Input: part model. Units: mm. Frame: model coordinates. Face numbers are marked on the shaded views. A direction names the side the tool comes from. Round coordinates to 2 decimals unless told otherwise and drop trailing zeros. Order: outer loops, then holes, each group sorted by start corner. A loop starts at its lowest first (then second) coordinate and runs counter-clockwise, first axis right, second up. Notation, with made-up numbers: M -6.5,-31.5 L 50.5,-31.5 A30 ccw 50.5,7.5 Z; hole C 46,17.25 d2. An arc over 180 degrees is marked long. One line per question, with ' | ' between items.
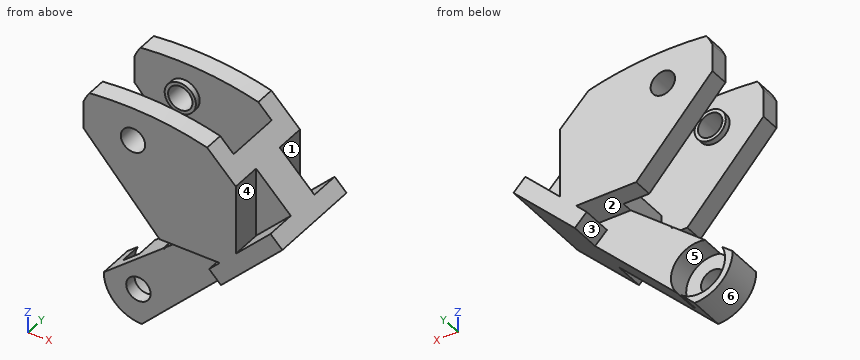
```python
from build123d import *

# Parameters (mm, degrees)
SKETCH_1_R           = 1.6
EXTRUDE_1_DEPTH      = 4.65
SKETCH_7_W           = 9
SKETCH_7_H           = 19
EXTRUDE_4_DEPTH      = 4
SKETCH_8_W           = 9
SKETCH_8_H           = 19
EXTRUDE_5_DEPTH      = 4
SKETCH_9_W           = 16
SKETCH_9_H           = 7.5
CUT_EXTRUDE_3_DEPTH  = 9
SKETCH_11_R          = 1.6
CUT_EXTRUDE_5_DEPTH  = 26.4
EXTRUDE_6_DEPTH      = 9
SKETCH_13_W          = 19
SKETCH_13_H          = 12.65
EXTRUDE_7_DEPTH      = 2
SKETCH_15_W          = 7.596607022
SKETCH_15_H          = 7.5
CUT_EXTRUDE_6_DEPTH  = 8
CUT_EXTRUDE_7_DEPTH  = 8
EXTRUDE_8_DEPTH      = 4.65
CUT_EXTRUDE_9_DEPTH  = 4.65
SKETCH_20_W          = 5.380169682
SKETCH_20_H          = 3
CUT_EXTRUDE_10_DEPTH = 7.5
CUT_EXTRUDE_11_DEPTH = 4.65
CUT_EXTRUDE_13_DEPTH = 13
CUT_EXTRUDE_15_DEPTH = 13
SKETCH_26_W          = 18.396488504
SKETCH_26_H          = 12.65
EXTRUDE_9_DEPTH      = 2.2
SKETCH_28_W          = 2.5
SKETCH_28_H          = 12.65
CUT_EXTRUDE_17_DEPTH = 18
CUT_EXTRUDE_18_DEPTH = 14
SKETCH_31_W          = 5
SKETCH_31_H          = 12.65
CUT_EXTRUDE_19_DEPTH = 20
SKETCH_32_R          = 3.55
CUT_EXTRUDE_20_DEPTH = 3
EXTRUDE_START        = 0.75
SKETCH_33_R          = 2.05
SKETCH_33_R_2        = 1.6
EXTRUDE_10_DEPTH     = 0.75
SKETCH_34_R          = 2.05
SKETCH_34_R_2        = 1.6
EXTRUDE_11_DEPTH     = 0.75


with BuildPart() as part:
    # 草图1 → 凸台-拉伸1 (new body)
    with BuildSketch(Plane(origin=(0, 0, 0), x_dir=(1, 0, 0), z_dir=(0, 1, 0))):
        with BuildLine():
            Line((5, 0), (20, 0))
            Line((20, 0), (20, -16))
            Line((20, -16), (9, -16))
            Line((9, -16), (9, -35))
            Line((9, -35), (0, -35))
            Line((0, -35), (0, -27))
            Line((0, -27), (0, -5))
            ThreePointArc((0, -5), (1.464466094, -1.464466094), (5, 0))
        make_face()
        with Locations(Location((4.55, -4.55, 0), (0, 0, 270))):
            Circle(SKETCH_1_R, mode=Mode.SUBTRACT)
    extrude(amount=EXTRUDE_1_DEPTH)

    # 草图7 → 凸台-拉伸4 (add)
    with BuildSketch(Plane(origin=(0, 4.65, 0), x_dir=(1, 0, 0), z_dir=(0, 1, 0))):
        with Locations((4.5, -25.5)):
            Rectangle(SKETCH_7_W, SKETCH_7_H)
    extrude(amount=EXTRUDE_4_DEPTH)

    # 草图8 → 凸台-拉伸5 (add)
    with BuildSketch(Plane.XZ):
        with Locations((4.5, 25.5)):
            Rectangle(SKETCH_8_W, SKETCH_8_H)
    extrude(amount=EXTRUDE_5_DEPTH)

    # 草图9 → 切除-拉伸3 (cut)
    with BuildSketch(Plane.ZY):
        with Locations((27, 2.325)):
            Rectangle(SKETCH_9_W, SKETCH_9_H)
    extrude(amount=-CUT_EXTRUDE_3_DEPTH, mode=Mode.SUBTRACT)

    # 草图11 → 切除-拉伸5 (cut)
    with BuildSketch(Plane(origin=(0, 8.65, 0), x_dir=(1, 0, 0), z_dir=(0, 1, 0))):
        with Locations(Location((6.5, -28, 0), (0, 0, 270))):
            Circle(SKETCH_11_R)
    extrude(amount=-CUT_EXTRUDE_5_DEPTH, mode=Mode.SUBTRACT)

    # 草图12 → 凸台-拉伸6 (add)
    with BuildSketch(Plane(origin=(9, 0, 0), x_dir=(0, 0, -1), z_dir=(1, 0, 0))):
        Polygon((-35, 8.65), (-35, 6.075), (-19, 6.075), (-19, -1.425), (-35, -1.425), (-35, -4), (-16, -4), (-16, 8.65), align=None)
    extrude(amount=EXTRUDE_6_DEPTH)

    # 草图13 → 凸台-拉伸7 (add)
    with BuildSketch(Plane(origin=(18, 0, 0), x_dir=(0, 0, -1), z_dir=(1, 0, 0))):
        with Locations((-25.5, 2.325)):
            Rectangle(SKETCH_13_W, SKETCH_13_H)
    extrude(amount=EXTRUDE_7_DEPTH)

    # 草图15 → 切除-拉伸6 (cut)
    with BuildSketch(Plane.ZY):
        with Locations((15.201696489, 2.325)):
            Rectangle(SKETCH_15_W, SKETCH_15_H)
    extrude(amount=-CUT_EXTRUDE_6_DEPTH, mode=Mode.SUBTRACT)

    # 草图16 → 切除-拉伸7 (cut)
    with BuildSketch(Plane(origin=(0, 4.65, 0), x_dir=(1, 0, 0), z_dir=(0, 1, 0))):
        Polygon((0, -5), (5.890898071, -11.403392978), (0, -11.403392978), align=None)
    extrude(amount=-CUT_EXTRUDE_7_DEPTH, mode=Mode.SUBTRACT)

    # 草图17 → 凸台-拉伸8 (add)
    with BuildSketch(Plane.XZ):
        with BuildLine():
            Line((20, 35), (20, 15))
            Line((20, 15), (31.064630957, 26.064630957))
            ThreePointArc((31.064630957, 26.064630957), (26.002686727, 31.114774273), (20, 35))
        make_face()
    extrude(amount=-EXTRUDE_8_DEPTH)

    # 草图19 → 切除-拉伸9 (cut)
    with BuildSketch(Plane(origin=(0, 4.65, 0), x_dir=(1, 0, 0), z_dir=(0, 1, 0))):
        Polygon((20, -15), (5, 0), (20, 0), align=None)
    extrude(amount=-CUT_EXTRUDE_9_DEPTH, mode=Mode.SUBTRACT)

    # 草图20 → 切除-拉伸10 (cut)
    with BuildSketch(Plane(origin=(0, -1.425, 0), x_dir=(1, 0, 0), z_dir=(0, 1, 0))):
        with Locations((10.690084841, -17.5)):
            Rectangle(SKETCH_20_W, SKETCH_20_H)
    extrude(amount=CUT_EXTRUDE_10_DEPTH, mode=Mode.SUBTRACT)

    # 草图21 → 切除-拉伸11 (cut)
    with BuildSketch(Plane.XZ):
        Polygon((13.380169682, 16), (0, 5), (8, 16), align=None)
    extrude(amount=-CUT_EXTRUDE_11_DEPTH, mode=Mode.SUBTRACT)

    # 草图22 → 切除-拉伸13 (cut)
    with BuildSketch(Plane(origin=(0, 8.65, 0), x_dir=(1, 0, 0), z_dir=(0, 1, 0))):
        Polygon((0, -16), (10, -16), (0, -27), align=None)
    extrude(amount=-CUT_EXTRUDE_13_DEPTH, mode=Mode.SUBTRACT)

    # 草图23 → 切除-拉伸15 (cut)
    with BuildSketch(Plane(origin=(0, 8.65, 0), x_dir=(1, 0, 0), z_dir=(0, 1, 0))):
        with BuildLine():
            Line((6.5, -35), (0, -35))
            Line((0, -35), (0, -30.598076211))
            ThreePointArc((0, -30.598076211), (2.574858823, -33.79596987), (6.5, -35))
        make_face()
    extrude(amount=-CUT_EXTRUDE_15_DEPTH, mode=Mode.SUBTRACT)

    # 草图26 → 凸台-拉伸9 (add)
    with BuildSketch(Plane(origin=(2.5, 0, -2.5), x_dir=(-0.7071067811865509, 0, -0.7071067811865442), z_dir=(0.7071067811865442, 0, -0.7071067811865509))):
        with Locations((-31.198244252, 2.325)):
            Rectangle(SKETCH_26_W, SKETCH_26_H)
    extrude(amount=-EXTRUDE_9_DEPTH)

    # 草图28 → 切除-拉伸17 (cut)
    with BuildSketch(Plane(origin=(2.5, 0, -2.5), x_dir=(-0.7071067811865509, 0, -0.7071067811865442), z_dir=(0.7071067811865442, 0, -0.7071067811865509))):
        with Locations((-39.646488504, 2.325)):
            Rectangle(SKETCH_28_W, SKETCH_28_H)
    extrude(amount=-CUT_EXTRUDE_17_DEPTH, mode=Mode.SUBTRACT)

    # 草图29 → 切除-拉伸18 (cut)
    with BuildSketch(Plane.XZ.offset(4)):
        with BuildLine():
            Line((29.650417395, 24.650417395), (19.300834789, 35))
            Line((19.300834789, 35), (1.773611639, 35))
            Line((1.773611639, 35), (0.803925841, 32.06875155))
            add(Edge.make_bspline(
                [(29.650417395, 24.650417395), (16.711479186, 33.756910479), (0.803925841, 32.06875155)],
                knots=[0, 0, 0, 1, 1, 1], degree=2))
        make_face()
    extrude(amount=-CUT_EXTRUDE_18_DEPTH, mode=Mode.SUBTRACT)

    # 草图31 → 切除-拉伸19 (cut)
    with BuildSketch(Plane(origin=(2.5, 0, -2.5), x_dir=(-0.7071067811865509, 0, -0.7071067811865442), z_dir=(0.7071067811865442, 0, -0.7071067811865509))):
        with Locations((-35.896488504, 2.325)):
            Rectangle(SKETCH_31_W, SKETCH_31_H)
    extrude(amount=-CUT_EXTRUDE_19_DEPTH, mode=Mode.SUBTRACT)

    # 草图32 → 切除-拉伸20 (cut)
    with BuildSketch(Plane(origin=(0, 4.65, 0), x_dir=(1, 0, 0), z_dir=(0, 1, 0))):
        with Locations((4.55, -4.55)):
            Circle(SKETCH_32_R)
    extrude(amount=-CUT_EXTRUDE_20_DEPTH, mode=Mode.SUBTRACT)

    # 草图33 → 凸台-拉伸10 (add)
    with BuildSketch(Plane(origin=(0, -1.425, 0), x_dir=(1, 0, 0), z_dir=(0, 1, 0)).offset(EXTRUDE_START)):
        with Locations(Location((6.5, -28, 0), (0, 0, 90))):
            Circle(SKETCH_33_R)
        with Locations(Location((6.5, -28, 0), (0, 0, 270))):
            Circle(SKETCH_33_R_2, mode=Mode.SUBTRACT)
    extrude(amount=-EXTRUDE_10_DEPTH)

    # 草图34 → 凸台-拉伸11 (add)
    with BuildSketch(Plane.XZ.offset(-6.075)):
        with Locations(Location((6.5, 28, 0), (0, 0, 270))):
            Circle(SKETCH_34_R)
        with Locations(Location((6.5, 28, 0), (0, 0, 90))):
            Circle(SKETCH_34_R_2, mode=Mode.SUBTRACT)
    extrude(amount=EXTRUDE_11_DEPTH)


solid = part.part
```
Item 1: First-contact query: pin 1 (2.5 mm diameter, centred on x = 15.5, y = 3, fed in from +Z); pin 2 (1.8 mm diameter, centred on x = 4.5, z = 4, fed in from +Y); pin 3 (11 mm diameter, centred on x = 11.5, z = 6, fed in from +Y); pin 4 (1 mm diameter, centred on y = 1.5, z = 18, fed in from -X). Flat tips, straight axial feed; report the tip coordinate or a pass-through.
Report:
pin 1: z = 19 | pin 2: through | pin 3: y = 4.65 | pin 4: x = 13.38
Item 2: Line query: line 1 along Y through (x, z) = (11.25, 22) (3 decimals); line 2 along Y through (x, z) = (7.5, 7); line 3 along X through (y, z) = (0.8, 4.55). Output: solid intervals per line, ascending. Write a range as from..to.
Report:
line 1: -4..-1.425, 6.075..8.65 | line 2: 0..4.65 | line 3: 0.02..2.95, 6.15..9.55
Item 3: Section query D-D, the plane z = 10. Return loops of the section in (x, y), plus the area to 3 significant figures.
Report:
outline: M 6.08,0 L 15,0 L 15,4.65 L 6.08,4.65 Z | area: 41.5 mm²
Item 4: Access query for the marked faces 1, 2 and 3. Directions: +Z, -Z, +X, -X, +Y, -Y. A direction counts if a zero-diameter tool reaches every point of the face in a straight line with its end or side. Return the directions, or none.
Report:
face 1: +Z, +Y | face 2: -X, +Y | face 3: -Z, -X, +Y
Item 5: Section query A-A, the plane z = 28. Return loops of the section in (x, y) (3 decimals).
Report:
outline: M 0,-4 L 4.9,-4 L 4.9,-0.675 L 4.45,-0.675 L 4.45,-1.425 L 0,-1.425 Z; M 0,6.075 L 4.45,6.075 L 4.45,5.325 L 4.9,5.325 L 4.9,8.65 L 0,8.65 Z; M 8.1,-4 L 19.23,-4 L 19.23,8.65 L 8.1,8.65 L 8.1,5.325 L 8.55,5.325 L 8.55,6.075 L 18,6.075 L 18,-1.425 L 8.55,-1.425 L 8.55,-0.675 L 8.1,-0.675 Z
Item 6: Section query C-C, the plane x = 22.75. Return loops of the section in (y, z).
Report:
outline: M -4,17.75 L 8.65,17.75 L 8.65,20.86 L 4.65,20.86 L 4.65,24.48 L 0,24.48 L 0,20.86 L -4,20.86 Z
Item 7: Mould query, pull axis Z, two halves, no side actions, for the marked faces 4, 5 and 6. Classes: +Z half, -Z half, draft (parallel to the pull), parting line (faces both ways), or undercut.
Report:
face 4: draft | face 5: undercut | face 6: -Z half
Item 8: Section query B-B, the plane z = 4.55. Return loops of the section in (x, y), plus the area to 3 significant figures.
Report:
outline: M 0.02,0 L 2.95,0 L 2.95,1.65 L 1,1.65 L 1,4.65 L 0.02,4.65 Z; M 6.15,0 L 9.55,0 L 9.55,4.65 L 8.1,4.65 L 8.1,1.65 L 6.15,1.65 Z | area: 17.7 mm²
